The figure shows three views and two pictorial views of one solid part (mm, origin at its lowest corner). Answer the questions. Round coordinates to 2 decimals unless told otherwise and drop trailing zeros. Order: outer loops, then holes, each group sorted by start corner. A loop starts at its lowest first (then second) coordinate and runs counter-clockwise, first axis right, second up. Notation, with made-up numbers: (13.5, -1.75) - (50.5, -1.75) arc R25 cw to (50.5, 11.25) - close; hole circle Ø6 at (6.25, -31.75). An arc over 180 degrees is marked (long way). Answer as a JSON object with one key per item and string values. Group by question number.
Q1. A cutting plane is placed at A-A on y = 12.5. Determine the outline of the cut face in (x, z).
Q2. A cutting plane is placed at B-B on x = 4. Determine the outline of the cut face in (y, z), and give its area (3 significant figures).
Q3. A cutting plane is placed at D-D on y = 3.25. Determine the outline of the cut face in (x, z).
Q4. Given pin 1 Ø10 at (x, z) = (6.5, 20.5) entering from -Y; pin 2 Ø5 at (x, z) = (13, 16.5) entering from -Y; pin 3 Ø2 at (y, z) = (16, 7) entering from +X; pin 4 Ø2 at (y, z) = (3, 12) entering from +X, each flat-ended and moving along its own axis, determine where each tip first touches the part or whether it passes through.
Q5. The mould has two halves that part along X. Classify the marked faces 1, 2, 3 and 4: pulls with the +X half, pulls with the -X half, needs draft (parallel to the pull), parting line crosses it, or undercut.
Q6. Consider line 1 (X direction, y = 4, z = 3.5); line 2 (X direction, y = 21, z = 3.1). Determine where each line is inside the solid, lowest interval first.
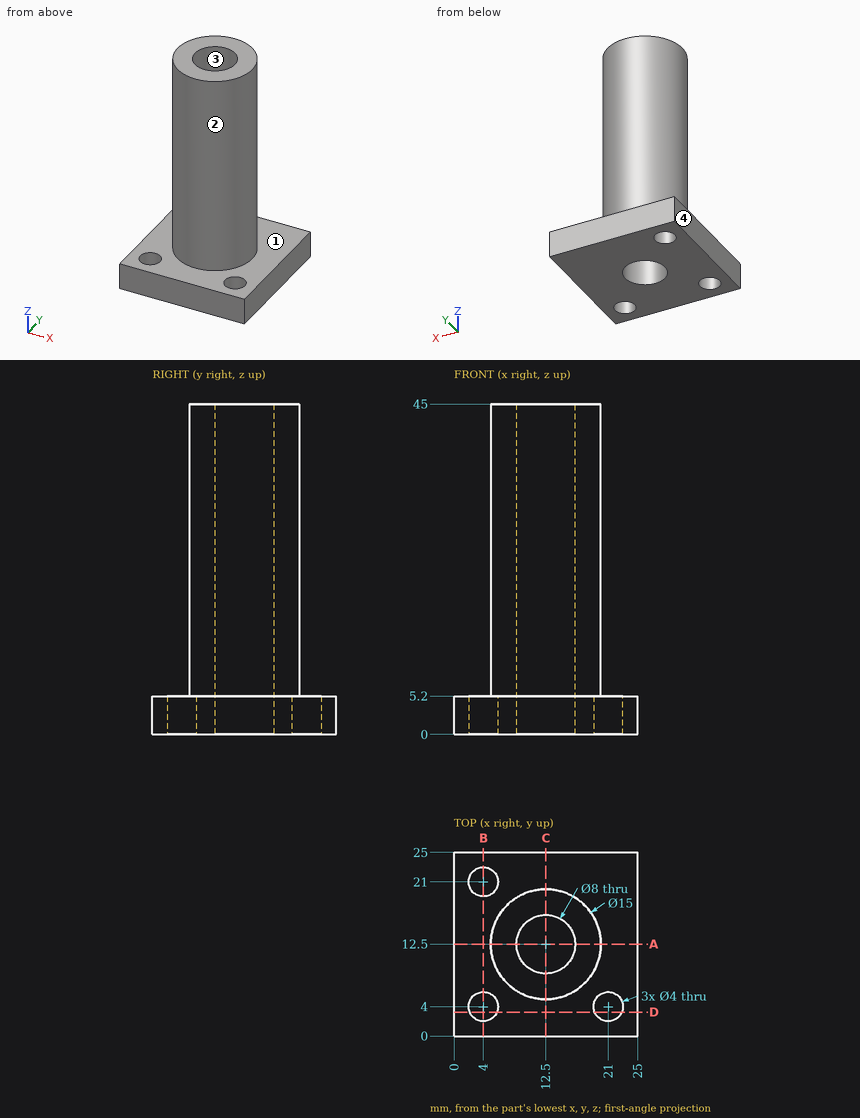
Result set:
{
 "1": {"outline": "(0, 0) - (8.5, 0) - (8.5, 45) - (5, 45) - (5, 5.2) - (0, 5.2) - close; (16.5, 0) - (25, 0) - (25, 5.2) - (20, 5.2) - (20, 45) - (16.5, 45) - close"},
 "2": {"outline": "(0, 0) - (2, 0) - (2, 5.2) - (0, 5.2) - close; (6, 0) - (19, 0) - (19, 5.2) - (6, 5.2) - close; (23, 0) - (25, 0) - (25, 5.2) - (23, 5.2) - close", "area": "88.4 mm²"},
 "3": {"outline": "(0, 0) - (2.15, 0) - (2.15, 5.2) - (0, 5.2) - close; (5.85, 0) - (19.15, 0) - (19.15, 5.2) - (5.85, 5.2) - close; (22.85, 0) - (25, 0) - (25, 5.2) - (22.85, 5.2) - close"},
 "4": {"pin 1": "stops at y = 5.07", "pin 2": "stops at y = 5", "pin 3": "stops at x = 19.57", "pin 4": "passes through"},
 "5": {"face 1": "needs draft", "face 2": "parting line crosses it", "face 3": "undercut", "face 4": "pulls with the -X half"},
 "6": {"line 1": "x = 0 to 2, 6 to 19, 23 to 25", "line 2": "x = 0 to 2, 6 to 25"}
}
